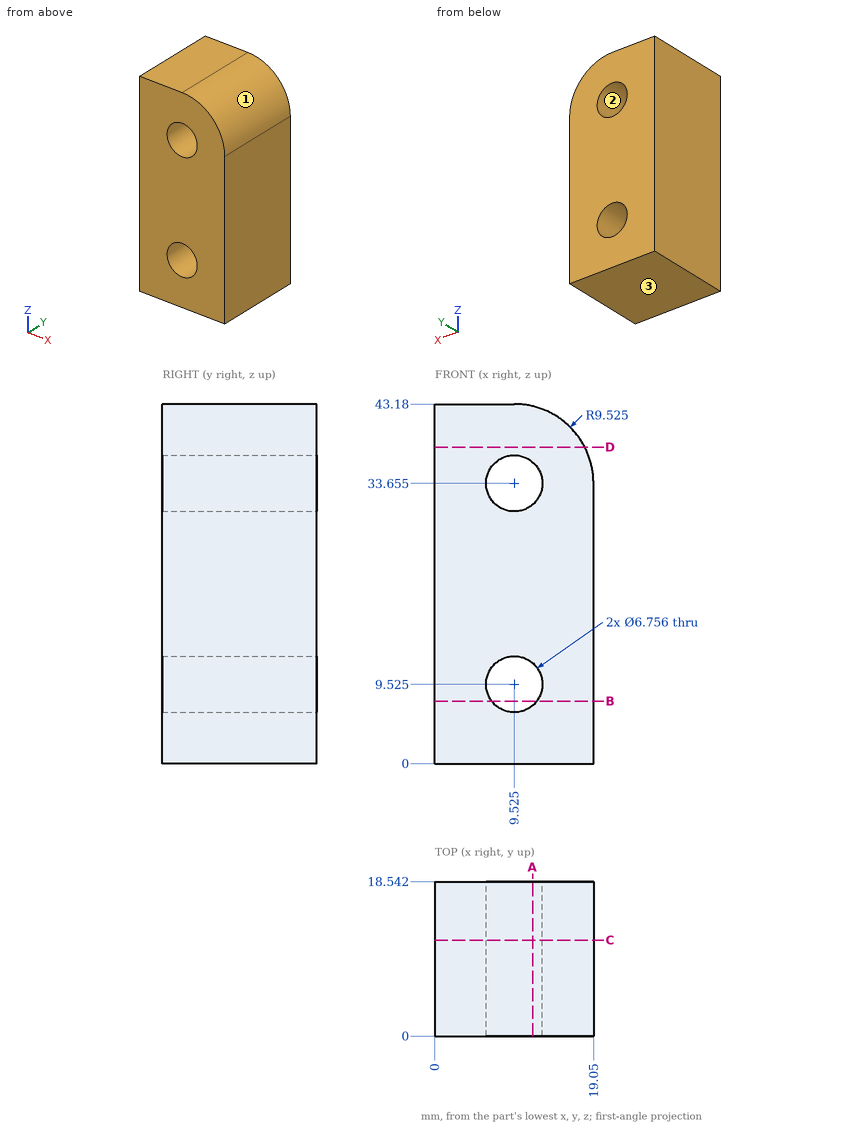
Geometry: see drawing. Coordinates: mm, zero at the bounding-box minimum. Give positions to 0.01 mm unless a question says otherwise; leave off trailing zeros. Order: outer loops, then holes, each group sorted by start corner. A loop starts at its lowest first (then second) coordinate and runs counter-clockwise, first axis right, second up. Notation, with made-up numbers: M 67,38 L 96,38 A33 cw 96,74 Z; hole C 72.5,-1.5 d9. An arc over 180 degrees is marked long. Answer as a JSON object with one key per item and string values.
1. Cut plane C-C, the plane y = 11.5. State how many separate pieces and enclosed holes the cut face has.
Result sheet:
{"separate pieces": "1", "enclosed holes": "2"}
2. Cut plane A-A, the plane x = 11.75. Output: boundary loops of the cut face in (y, z), and give its area (3 significant figures).
Result sheet:
{"outline": "M 0,0 L 18.54,0 L 18.54,6.98 L 0,6.98 Z; M 0,12.07 L 18.54,12.07 L 18.54,31.11 L 0,31.11 Z; M 0,36.2 L 18.54,36.2 L 18.54,42.92 L 0,42.92 Z", "area": "607 mm²"}
3. First-contact query: P1, Ø1.5, axis at x = 15, y = 13, coming from the +Z side (1 decimal). Flat tip, straight axial feed; report the tip coordinate or a pass-through.
Result sheet:
{"P1": "z = 41.9"}
4. Cut plane D-D, the plane z = 38. Output: boundary loops of the cut face in (x, y).
Result sheet:
{"outline": "M 0,0 L 18,0 L 18,18.54 L 0,18.54 Z"}
5. Ray query, line 1 (Z direction, x = 10.5, y = 8.5); line 2 (Z direction, x = 8.25, y = 6.5); line 3 (X direction, y = 9.25, z = 36) (1 decimal). Return the intervals inside material, ascending. Write a range as [from, to].
Result sheet:
{"line 1": "[0, 6.29], [12.76, 30.42], [36.89, 43.13]", "line 2": "[0, 6.4], [12.65, 30.53], [36.78, 43.18]", "line 3": "[0, 7.1], [12, 18.8]"}
6. Pull-direction query (X, two-part tool) for the marked faces 1, 2 and 3; classes: +X half, -X half, draft (parallel to the pull), parting line (faces both ways), or undercut.
Result sheet:
{"face 1": "+X half", "face 2": "undercut", "face 3": "draft"}
7. Cut plane B-B, the plane z = 7.5. Output: boundary loops of the cut face in (x, y).
Result sheet:
{"outline": "M 0,0 L 6.82,0 L 6.82,18.54 L 0,18.54 Z; M 12.23,0 L 19.05,0 L 19.05,18.54 L 12.23,18.54 Z"}
